from build123d import *

# Parameters (mm, degrees)
SALIENTE_EXTRUIR1_DEPTH = 90
CROQUIS2_OUTSIDE_W      = 35.078
CROQUIS2_OUTSIDE_H      = 33.302
CROQUIS2_OUTSIDE_R      = 4.75
CORTAR_EXTRUIR1_DEPTH   = 9.525


with BuildPart() as part:
    # Croquis1 → Saliente-Extruir1 (new body)
    with BuildSketch(Plane(origin=(0, 0, 0), x_dir=(1, 0, 0), z_dir=(0, 1, 0))):
        Polygon((3.502287207, -6.44184117), (7.329941703, -0.187850892), (3.827654496, 6.253990277), (-3.502287207, 6.44184117), (-7.329941703, 0.187850892), (-3.827654496, -6.253990277), align=None)
    extrude(amount=SALIENTE_EXTRUIR1_DEPTH)

    # Croquis2 outside → Cortar-Extruir1 (cut)
    with BuildSketch(Plane.XZ):
        Rectangle(CROQUIS2_OUTSIDE_W, CROQUIS2_OUTSIDE_H)
        with Locations(Location((0, 0, 0), (0, 0, 270))):
            Circle(CROQUIS2_OUTSIDE_R, mode=Mode.SUBTRACT)
    extrude(amount=-CORTAR_EXTRUIR1_DEPTH, mode=Mode.SUBTRACT)


solid = part.part
Check sheet for the modelled part. Datum: model origin and axes. Units: mm. A direction names the side the tool comes from. Give positions to 0.01 mm unless a question says otherwise; leave off trailing zeros. Loops run counter-clockwise (first coordinate to the right, second up) from the corner with the lowest first, then second, coordinate; pieces in that order, holes last. Notation, with made-up numbers: M -19,-1 L 32,-1 A28 cw 32,18 Z; hole C 70.5,6.5 d6. An arc over 180 degrees is marked long. Answer as a JSON object with one key per item and string values. Group by question number.
Q1. Access from +Z, -Z, +X, -X, +Y, -Y to the whole of each face (thin tool, end or side, straight path). Record for faces 1 (the flat face through (5, 9.525, 0)), 2 (the flat face through (5.39, 49.2, 3.36)).
Q2. Go/stop test with flat-tipped pins: P1, Ø5, axis at x = 4.5, y = 55.5, coming from the +Z side; P2, Ø1, axis at x = 5.5, z = 0, coming from the -Y side (3 decimals); P3, Ø8, axis at x = -4.5, y = 60.5, coming from the +Z side; P4, Ø1, axis at y = 39.5, z = -0.5, coming from the +X side. Record where each tip stops, or that it passes through.
Q3. Material ranges on line 1 along Y through (x, z) = (5, 1.25) (3 decimals); line 2 along Z through (x, y) = (6.75, 43); line 3 along X through (y, z) = (66, -4), recorded low to high. Write a range as [from, to].
Q4. Cross-section at D-D on x = 2.25. Record the cut outline in (y, z) (3 decimals).
Q5. Cross-section at A-A on x = -1.75. Record the cut outline in (y, z) (3 decimals).
Q6. Cross-section at C-C on z = -5.5. Record the cut outline in (x, y) (3 decimals), then the cut area to 3 significant figures.
Q7. Cross-section at B-B on y = 49. Record the cut outline in (x, z).
Evaluation:
{
 "1": {"face 1": "-Y", "face 2": "+Z, +X, +Y, -Y"},
 "2": {"P1": "stops at z = 6.44", "P2": "stops at y = 9.525", "P3": "stops at z = 6.34", "P4": "stops at x = 7.23"},
 "3": {"line 1": "y = [9.525, 90]", "line 2": "z = [-0.88, 1.14]", "line 3": "x = [-5, 5.05]"},
 "4": {"outline": "M 0,-4.183 L 9.525,-4.183 L 9.525,-6.294 L 90,-6.294 L 90,6.41 L 9.525,6.41 L 9.525,4.183 L 0,4.183 Z"},
 "5": {"outline": "M 0,-4.416 L 9.525,-4.416 L 9.525,-6.397 L 90,-6.397 L 90,6.307 L 9.525,6.307 L 9.525,4.416 L 0,4.416 Z"},
 "6": {"outline": "M -4.079,9.525 L 4.238,9.525 L 4.238,90 L -4.079,90 Z", "area": "669 mm2"},
 "7": {"outline": "M -7.33,-0.19 L -3.5,-6.44 L 3.83,-6.25 L 7.33,0.19 L 3.5,6.44 L -3.83,6.25 Z"}
}
